Source: CAD feature listing. Evaluate the final solid. Frame: model axes, mm. A direction names the side the tool comes from. Round coordinates to 2 decimals unless told otherwise and drop trailing zeros. Write each loop counter-clockwise with the first axis right and the second up, starting at its lowest first coordinate (ties: lowest second). Pieces come first, ordered by that corner, then holes.
from build123d import *

# Parameters (mm, degrees)
F1_DEPTH    = 12.7
F2_W        = 9.5430067153
F2_H        = 12.7
F3_DEPTH    = 7.62
F4_R        = 2.54
F5_DEPTH    = 12.7
F6_R        = 5.08
F7_T1_DEPTH = 35.8885048544


# Not quite as in the source:
# - a fillet or chamfer that OpenCascade refuses, or shapes differently, is made with other operations: its cross-section is extruded or revolved along the edge and cut away or added


with BuildPart() as f1:
    # F0 (on Front) → F1 (new body)
    with BuildSketch(Plane.XZ):
        with BuildLine():
            Line((-21.0839635167, 28.5975757856), (-30.6269058684, 28.632624914))
            ThreePointArc((-30.6269058684, 28.632624914), (-40.6992100974, -1.826971115), (-30.8592707303, -32.3624242144))
            Line((-30.8592707303, -32.3624242144), (-21.2263563985, -32.3624242144))
            ThreePointArc((-21.2263563985, -32.3624242144), (-33.1531180249, -1.8543988892), (-21.0839635167, 28.5975757856))
        make_face()
        Polygon((-21.2263563985, -32.3624242144), (-30.8592707303, -32.3624242144), (-35.6757278961, -32.3624242144), (-35.6757278961, -38.7124242144), (-21.2263563985, -38.7124242144), align=None)
        with BuildLine():
            Line((-35.6757278961, -38.7124242144), (-35.6757278961, -32.3624242144))
            ThreePointArc((-35.6757278961, -32.3624242144), (-38.8507278961, -35.5374242144), (-35.6757278961, -38.7124242144))
        make_face()
    extrude(amount=F1_DEPTH)

    # F2 (on face) → F3 (join)
    with BuildSketch(Plane(origin=(0.1047467849, 0, 28.519754313), x_dir=(0.9999932554, 0, -0.0036727553), z_dir=(0.0036727553, 0, 0.9999932554))):
        with Locations((-25.9603565693, -6.35)):
            Rectangle(F2_W, F2_H)
    extrude(amount=F3_DEPTH)

    # F4 (on face) → F5 (join)
    with BuildSketch(Plane(origin=(-21.1887103016, 0, 0.0778214726), x_dir=(0, 1, 0), z_dir=(0.9999932554, 0, -0.0036727553))):
        with Locations((-6.35, 32.2985388339)):
            Circle(F4_R)
    extrude(amount=F5_DEPTH)

    # F6
    f6_edges = [f1.edges().sort_by_distance(p)[0] for p in [
        (-21.226356, -6.35, -38.712424),
    ]]
    fillet(f6_edges, radius=F6_R)

    # F7: fillet of radius 30.8120471725 on 1 edges, made by hand

    # F7_s2 → F7_t1 (cut)
    with BuildSketch(Plane.XZ.offset(-11.5942524272)):
        with BuildLine():
            ThreePointArc((-21.2263563985, -33.6324242144), (-22.6013772134, -31.1490637357), (-24.1991044236, -28.8027838569))
            ThreePointArc((-24.1991044236, -28.8027838569), (-22.7589105371, -30.6211702571), (-21.2263563985, -32.3624242144))
            Line((-21.2263563985, -32.3624242144), (-21.2263563985, -33.6324242144))
        make_face()
    extrude(amount=F7_T1_DEPTH, mode=Mode.SUBTRACT)


solid = f1.part
1) Section query D-D on y = -6.75. Return the cut outline in (x, z) (3 decimals).
Taken from the geometry:
outline: (-35.676, -38.712) - (-26.306, -38.712) arc R5.08 ccw to (-21.226, -33.632) arc R30.812 ccw to (-24.199, -28.803) arc R44.715 cw to (-21.084, 28.598) - (-21.079, 29.868) - (-8.379, 29.821) - (-8.361, 34.838) - (-21.061, 34.884) - (-21.056, 36.218) - (-30.599, 36.253) - (-30.627, 28.633) arc R51.688 ccw to (-30.859, -32.362) - (-35.676, -32.362) arc R3.175 ccw to start
2) Material intervals for line 1 (Z direction, x = -22.5, y = -8); line 2 (Z direction, x = -25, y = -9.25); line 3 (X direction, y = -4.75, z = 29.5), sorted ascending.
Taken from the geometry:
line 1: z = -37 to -31.31, 27.01 to 36.22
line 2: z = -38.54 to -27.7, 23.78 to 36.23
line 3: x = -30.62 to -21.08
3) Section query C-C on x = -37.5. Return the cut outline in (y, z), then the cut area to 3 significant figures.
Taken from the geometry:
outline: (-12.7, -38.14) - (0, -38.14) - (0, -32.94) - (-12.7, -32.94) - close; (-12.7, -19.93) - (0, -19.93) - (0, 15.88) - (-12.7, 15.88) - close
area: 521 mm2
4) Section query A-A on x = -29. Return the cut outline in (y, z), then the cut area to 3 significant figures.
Taken from the geometry:
outline: (-12.7, -38.71) - (0, -38.71) - (0, -20.78) - (-12.7, -20.78) - close; (-12.7, 16.86) - (0, 16.86) - (0, 36.25) - (-12.7, 36.25) - close
area: 474 mm2
5) Contact query for flat-ended pins moving along their axis: P1, Ø4, axis at y = -6, z = -21, coming from the -X side; P2, Ø4, axis at x = -22.5, y = -7.5, coming from the -Z side; P3, Ø2, axis at y = -4.5, z = -5, coming from the -X side. Output: stop coordinate, or through.
Taken from the geometry:
P1: stops at x = -37.83
P2: stops at z = -38.38
P3: stops at x = -40.66
6) Reachability of faces 1 (the face through (-35, 0, -2)), 2 (the face through (-22.581, -6.261, -31.183)), 3 (the face through (-33, -6, -32.362)) from +Z, -Z, +X, -X, +Y, -Y: full face, straight path, thin tool, end or side. Return the list, or none.
Taken from the geometry:
face 1: +Z, -Z, +X, -X, +Y
face 2: +X, +Y, -Y
face 3: -X, +Y, -Y
7) Section query B-B on y = -2.5. Return the cut outline in (x, z) (3 decimals), then the cut area to 3 significant figures.
Taken from the geometry:
outline: (-35.676, -38.712) - (-26.306, -38.712) arc R5.08 ccw to (-21.226, -33.632) arc R30.812 ccw to (-24.199, -28.803) arc R44.715 cw to (-21.084, 28.598) - (-21.056, 36.218) - (-30.599, 36.253) - (-30.627, 28.633) arc R51.688 ccw to (-30.859, -32.362) - (-35.676, -32.362) arc R3.175 ccw to start
area: 669 mm2
